```python
from build123d import *

# Parameters (mm, degrees)
F0_R             = 37.5
F1_DEPTH         = 16
F3_START         = -11.4
F2_R             = 12.8
F3_DEPTH         = 28.6
F4_R             = 7.75
F5_DEPTH         = 14
F12_COPIES_COUNT = 3
F12_COPIES_ANGLE = 90


# Not quite as in the source:
# - a pattern or mirror of a feature is missing from the dataset's text; its kind, count and spacing are read off the source's solid


with BuildPart() as f1:
    # F0 (on Top) → F1 (new body)
    with BuildSketch(Plane.XY):
        Circle(F0_R)
    extrude(amount=F1_DEPTH)

    # F2 (on Right) → F3 (cut)
    with BuildSketch(Plane.YZ.offset(F3_START)):
        with Locations((0, 8)):
            Circle(F2_R)
    extrude(amount=-F3_DEPTH, mode=Mode.SUBTRACT)

    # F4 (on face) → F5 (cut)
    with BuildSketch(Plane.XY.offset(16)):
        Circle(F4_R)
    extrude(amount=-F5_DEPTH, mode=Mode.SUBTRACT)

    # F7 (on Front) → F8 (revolve)
    with BuildSketch(Plane.XZ):
        Polygon((0, 2), (0, 4.4), (-2.2, 4.4), (-4.6, 2), align=None)
    revolve(axis=Axis((0, 0, 3.2), (0, 0, 1)))

    # F9 (on Front) → F10 (revolve, cut)
    with BuildSketch(Plane.XZ):
        with BuildLine():
            ThreePointArc((0, -10), (4.7376154339, -8.0376154339), (6.7, -3.3))
            ThreePointArc((6.7, -3.3), (4.7376154339, 1.4376154339), (0, 3.4))
            Line((0, 3.4), (0, -10))
        make_face()
    revolve(axis=Axis((0, 0, -3.3), (0, 0, -1)), mode=Mode.SUBTRACT)

    # F11 (on offset) → F12 (revolve, cut)
    with BuildSketch(Plane.XY.offset(8)):
        with BuildLine():
            Line((16, 0), (52, 0))
            Line((52, 0), (52, 5.15))
            Line((52, 5.15), (21.15, 5.15))
            ThreePointArc((21.15, 5.15), (17.5084000769, 3.6415999231), (16, 0))
        make_face()
    f12 = revolve(axis=Axis((34, 0, 8), (1, 0, 0)), mode=Mode.SUBTRACT)

    # F12_copies: F12 ×3 about axis
    f12_copies_axis = Axis((0, 0, 0), (0, 0, -1))
    for i in range(1, F12_COPIES_COUNT):
        add(f12.rotate(f12_copies_axis, i * F12_COPIES_ANGLE / (F12_COPIES_COUNT - 1)), mode=Mode.SUBTRACT)


solid = f1.part
```
Could you check a few things on this model? Use its own coordinates, in mm. A direction names the side the tool comes from. Coordinates: 2 decimals unless noted, no trailing zeros. Write each loop counter-clockwise with the first axis right and the second up, starting at its lowest first coordinate (ties: lowest second). Pieces come first, ordered by that corner, then holes. Notation, with made-up numbers: (87.5, -3) -> (108.5, -3) arc R22 ccw to (108.5, 28) -> close; hole circle Ø11 at (61.5, -39.75). An arc over 180 degrees is marked (long way). One line per question, with ' | ' between items. Start each with the question number.
1. If we section it at D-D (x = 0): Please give me the cut outline in (y, z).
2. If we section it at B-B (z = 11.5): Please give me the cut outline in (x, y).
3. For faces 4 (the face through (29.211, -1.116, 2.972)), 5 (the face through (-23.6, -12.8, 8.1)), 6 (the face through (0, 0, 4.4)), which set-ups out of +Z, -Z, +X, -X, +Y, -Y let a thin tool reach every point of the face, with its end or its side?
4. Please list where these lines run through material, in increasing order: line 1 along Z through (x, y) = (0, -32.25); line 2 along X through (y, z) = (-18, 8.5); line 3 along X through (y, z) = (-1, 2.25).
5. If we section it at C-C (y = 0): Please give me the cut outline in (x, z), and give its area (3 significant figures).
6. If we section it at A-A (x = -30): Please give me the cut outline in (y, z), and give its area (3 significant figures).
7. Will these pins go through, and if not, where does the flat tip stop? P1, Ø1.5, axis at y = 1.5, z = 13.5, coming from the -X side; P2, Ø2, axis at x = 3, z = 8.5, coming from the -Y side; P3, Ø4, axis at x = -15, z = 8.5, coming from the -Y side.
8. Thinking about a two-plate mould opening in Z: for faces 1 (the face through (-1.116, -29.211, 2.972)), 2 (the face through (-2.24, -0.71, 4.25)), 3 (the face through (-1.009, 7.684, 9.098)), which applies, pulls with the +Z half, pulls with the -Z half, needs draft (parallel to the pull), parting line crosses it, or undercut?
Return value:
1) outline: (-37.5, 0) -> (-5.83, 0) arc R6.7 cw to (5.83, 0) -> (37.5, 0) -> (37.5, 16) -> (7.75, 16) -> (7.75, 2) -> (4.6, 2) -> (2.2, 4.4) -> (-2.2, 4.4) -> (-4.6, 2) -> (-7.75, 2) -> (-7.75, 16) -> (-37.5, 16) -> (-37.5, 13.15) -> (-21.15, 13.15) arc R5.15 cw to (-21.15, 2.85) -> (-37.5, 2.85) -> close
2) outline: (-35.42, -12.31) arc R37.5 ccw to (-3.78, -37.31) -> (-3.78, -21.15) arc R3.78 cw to (3.78, -21.15) -> (3.78, -37.31) arc R37.5 ccw to (23.71, -29.05) -> (12.28, -17.63) arc R3.78 cw to (17.63, -12.28) -> (29.05, -23.71) arc R37.5 ccw to (37.31, -3.78) -> (21.15, -3.78) arc R3.78 cw to (21.15, 3.78) -> (37.31, 3.78) arc R37.5 ccw to (-35.42, 12.31) -> (-11.4, 12.31) -> (-11.4, -12.31) -> close; hole circle Ø15.5 at (0, 0)
3) face 4: +X | face 5: -X | face 6: +Z
4) line 1: z = 0 to 2.85, 13.15 to 16 | line 2: x = -32.9 to -4.04, 4.04 to 10.83, 25.25 to 32.9 | line 3: x = -11.4 to -7.69, -4.23 to -3.62, 3.62 to 4.23, 7.69 to 37.49
5) outline: (-11.4, 0) -> (-5.83, 0) arc R6.7 cw to (5.83, 0) -> (37.5, 0) -> (37.5, 2.85) -> (21.15, 2.85) arc R5.15 cw to (21.15, 13.15) -> (37.5, 13.15) -> (37.5, 16) -> (7.75, 16) -> (7.75, 2) -> (4.6, 2) -> (2.2, 4.4) -> (-2.2, 4.4) -> (-4.6, 2) -> (-7.75, 2) -> (-7.75, 16) -> (-11.4, 16) -> close | area: 344 mm²
6) outline: (-22.5, 0) -> (-9.99, 0) arc R12.8 cw to (-9.99, 16) -> (-22.5, 16) -> close; (9.99, 0) -> (22.5, 0) -> (22.5, 16) -> (9.99, 16) arc R12.8 cw to start | area: 339 mm²
7) P1: stops at x = -11.4 | P2: stops at y = -17.96 | P3: stops at y = -35.17
8) face 1: undercut | face 2: pulls with the +Z half | face 3: needs draft
